Geometry: final body of the model. Coordinates: model frame, mm. Face numbers are marked on the shaded views. A direction names the side the tool comes from. Give positions to 0.01 mm unless a question says otherwise; leave off trailing zeros. Order: outer loops, then holes, each group sorted by start corner. A loop starts at its lowest first (then second) coordinate and runs counter-clockwise, first axis right, second up. Notation, with made-up numbers: (63.5, 1) -> (107.5, 1) arc R19 ccw to (107.5, 28) -> close; hole circle Ø10 at (-15.5, -30). An arc over 180 degrees is marked (long way). Answer in a Markdown table with one row per item. Add a question column.
Q1. Cut plane C-C on x = 0. Return the cut outline in (y, z).
Q2. Contact query for flat-ended pins moving along their axis: P1, Ø1.5, axis at x = -19, y = 11.5, coming from the -Z side; P2, Ø1.5, axis at x = 2.5, y = 11.5, coming from the +Z side; P3, Ø6, axis at x = -18.5, y = 4.5, coming from the +Z side. Output: stop coordinate, or through.
Q3. Cut plane B-B on z = 0. Return the cut outline in (x, y), and give its area (3 significant figures).
Q4. Cut plane A-A on y = 4. Return the cut outline in (x, z).
Q5. Pull-direction query (Y, two-part tool) for the marked faces 1, 2 and 3; classes: +Y half, -Y half, draft (parallel to the pull), parting line (faces both ways), or undercut.
Q6. Cut plane D-D on z = -15. Return the cut outline in (x, y).
Q7. Set-up query: the marked faces 4 and 5. Return all of +Z, -Z, +X, -X, +Y, -Y with unobstructed straight access to the full face (end or side cutting, diameter ignored); none if empty.
Q8. Line query: line 1 along X through (y, z) = (9, 0); line 2 along Z through (x, y) = (0.5, 11.25); line 3 along Y through (x, z) = (6, 13). Output: solid intervals per line, ascending. Write a range as from..to.
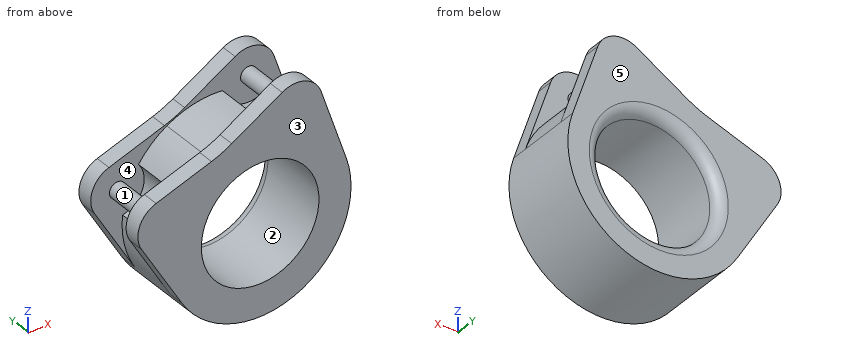
from build123d import *

# Parameters (mm, degrees)
SKETCH1_R               = 17
SKETCH1_R_2             = 11
BOSS_EXTRUDE1_DEPTH     = 15
BOSS_EXTRUDE2_START     = -15
BOSS_EXTRUDE2_DEPTH     = 15
FILLET1_R               = 5
CUT_EXTRUDE1_START      = -12
SKETCH3_R               = 1.5
CUT_EXTRUDE1_DEPTH      = 9
CIRPATTERN1_START       = 3
CIRPATTERN1_DEPTH       = 9
CIRPATTERN1_2_DEPTH     = 3
CIRPATTERN1_START_2     = 12
CIRPATTERN1_3_DEPTH     = 3
CIRPATTERN1_4_OUTLINE_R = 1.5
CIRPATTERN1_4_DEPTH     = 9
FILLET2_R               = 20
FILLET3_R               = 2


# Read off the part's stored shape, not the designer's step: CirPattern1
with BuildPart() as part:
    # Sketch1 → Boss-Extrude1 (new body)
    with BuildSketch(Plane(origin=(0, 0, 0), x_dir=(1, 0, 0), z_dir=(0, 1, 0))):
        with Locations(Location((0, 0, 0), (0, 0, 270))):
            Circle(SKETCH1_R)
        with Locations(Location((0, 0, 0), (0, 0, 270))):
            Circle(SKETCH1_R_2, mode=Mode.SUBTRACT)
    extrude(amount=BOSS_EXTRUDE1_DEPTH)

    # Sketch2 → Boss-Extrude2 (add)
    with BuildSketch(Plane(origin=(0, 15, 0), x_dir=(1, 0, 0), z_dir=(0, 1, 0)).offset(BOSS_EXTRUDE2_START)):
        with BuildLine():
            Line((-8.632611981, -14.645067784), (9.437831165, -25.296785229))
            Line((9.437831165, -25.296785229), (16.115556306, -5.411916938))
            ThreePointArc((16.115556306, -5.411916938), (5.942338141, -15.927605514), (-8.632611981, -14.645067784))
        make_face()
    extrude(amount=BOSS_EXTRUDE2_DEPTH)

    # Fillet1
    fillet1_edges = [part.edges().sort_by_distance(p)[0] for p in [
        (9.437831165, 7.5, 25.296785229),
    ]]
    fillet(fillet1_edges, radius=FILLET1_R)

    # Sketch3 → Cut-Extrude1 (cut)
    with BuildSketch(Plane(origin=(0, 15, 0), x_dir=(1, 0, 0), z_dir=(0, 1, 0)).offset(CUT_EXTRUDE1_START)):
        with BuildLine():
            ThreePointArc((1.752523284, -16.909425246), (-3.621565103, -16.609764183), (-8.632611981, -14.645067784))
            Line((-8.632611981, -14.645067784), (4.122994946, -22.163927157))
            ThreePointArc((4.122994946, -22.163927157), (8.409744981, -22.541144136), (11.401867971, -19.448294555))
            Line((11.401867971, -19.448294555), (16.115556306, -5.411916938))
            ThreePointArc((16.115556306, -5.411916938), (13.615928399, -10.178727515), (9.751380337, -13.925177971))
            ThreePointArc((9.751380337, -13.925177971), (4.914251957, -13.171964422), (1.752523284, -16.909425246))
        make_face()
        with Locations(Location((6.661998469, -17.856554279, 0), (0, 0, 270))):
            Circle(SKETCH3_R, mode=Mode.SUBTRACT)
    extrude(amount=CUT_EXTRUDE1_DEPTH, mode=Mode.SUBTRACT)

    # CirPattern1 outline → CirPattern1 (cut)
    with BuildSketch(Plane(origin=(0, 0, 0), x_dir=(1, 0, 0), z_dir=(0, 1, 0)).offset(CIRPATTERN1_START)):
        with BuildLine():
            ThreePointArc((-13.925177971, -9.751380337), (-13.171964422, -4.914251957), (-16.909425246, -1.752523284))
            ThreePointArc((-16.909425246, -1.752523284), (-15.927605515, -5.942338141), (-13.925177971, -9.751380337))
        make_face()
    extrude(amount=CIRPATTERN1_DEPTH, mode=Mode.SUBTRACT)

    # CirPattern1 2 outline → CirPattern1 2 (add)
    with BuildSketch(Plane(origin=(0, 0, 0), x_dir=(1, 0, 0), z_dir=(0, 1, 0))):
        with BuildLine():
            Line((-14.645067784, 8.632611981), (-22.163927157, -4.122994946))
            ThreePointArc((-22.163927157, -4.122994946), (-22.541144136, -8.409744981), (-19.448294555, -11.401867971))
            Line((-19.448294555, -11.401867971), (-7.099245913, -15.548918451))
            Line((-7.099245913, -15.548918451), (-8.632611981, -14.645067784))
            ThreePointArc((-8.632611981, -14.645067784), (-16.459805212, -4.25144827), (-14.645067784, 8.632611981))
        make_face()
    extrude(amount=CIRPATTERN1_2_DEPTH)

    # CirPattern1 3 outline → CirPattern1 3 (add)
    with BuildSketch(Plane(origin=(0, 0, 0), x_dir=(1, 0, 0), z_dir=(0, 1, 0)).offset(CIRPATTERN1_START_2)):
        with BuildLine():
            Line((-14.645067784, 8.632611981), (-22.163927157, -4.122994946))
            ThreePointArc((-22.163927157, -4.122994946), (-22.541144136, -8.409744981), (-19.448294555, -11.401867971))
            Line((-19.448294555, -11.401867971), (-7.099245913, -15.548918451))
            Line((-7.099245913, -15.548918451), (-8.632611981, -14.645067784))
            ThreePointArc((-8.632611981, -14.645067784), (-16.459805212, -4.25144827), (-14.645067784, 8.632611981))
        make_face()
    extrude(amount=CIRPATTERN1_3_DEPTH)

    # CirPattern1 4 outline → CirPattern1 4 (add)
    with BuildSketch(Plane(origin=(0, 0, 0), x_dir=(1, 0, 0), z_dir=(0, 1, 0)).offset(CIRPATTERN1_START)):
        with Locations((-17.856554279, -6.661998469)):
            Circle(CIRPATTERN1_4_OUTLINE_R)
    extrude(amount=CIRPATTERN1_4_DEPTH)

    # Fillet2
    fillet2_edges = [part.edges().sort_by_distance(p)[0] for p in [
        (-7.099245913, 13.5, 15.548918451),
        (-7.099245913, 1.5, 15.548918451),
    ]]
    fillet(fillet2_edges, radius=FILLET2_R)

    # Fillet3
    fillet3_edges = [part.edges().sort_by_distance(p)[0] for p in [
        (0, 15, -11),
    ]]
    fillet(fillet3_edges, radius=FILLET3_R)


solid = part.part
Completed:
| question | item | result |
|---|---|---|
| 1 | outline | (0, -17) -> (15, -17) -> (15, -13) arc R2 ccw to (13, -11) -> (0, -11) -> close; (0, 11) -> (13, 11) arc R2 ccw to (15, 13) -> (15, 19.73) -> (12, 19.73) -> (12, 17) -> (3, 17) -> (3, 19.73) -> (0, 19.73) -> close |
| 2 | P1 | stops at z = -2.19 |
| 2 | P2 | stops at z = 21.54 |
| 2 | P3 | stops at z = 12.59 |
| 3 | outline | (-19.73, 0) -> (-11, 0) -> (-11, 13) arc R2 ccw to (-13, 15) -> (-19.73, 15) -> (-19.73, 12) -> (-17, 12) -> (-17, 3) -> (-19.73, 3) -> close; (11, 0) -> (17, 0) -> (17, 15) -> (13, 15) arc R2 ccw to (11, 13) -> close |
| 3 | area | 195 mm² |
| 4 | outline | circle Ø3 at (-17.86, 6.66); (-16.91, 1.75) arc R17 ccw (long way) to (9.75, 13.93) arc R5 cw to (1.75, 16.91) arc R17 ccw to (-13.93, 9.75) arc R5 cw to start; circle Ø3 at (6.66, 17.86); hole circle Ø22 at (0, 0) |
| 5 | face 1 | undercut |
| 5 | face 2 | draft |
| 5 | face 3 | -Y half |
| 6 | outline | (-8, 0) -> (8, 0) -> (8, 15) -> (-8, 15) -> close |
| 7 | face 4 | none |
| 7 | face 5 | +Z, -Z, +X, -X, +Y |
| 8 | line 1 | x = -17..-11, 11..17 |
| 8 | line 2 | z = -16.99..-10.99, 10.99..16.99 |
| 8 | line 3 | y = 0..3, 12..15 |
